Check sheet for the modelled part. Datum: model origin and axes. Units: mm. A direction names the side the tool comes from. Give positions to 0.01 mm unless a question says otherwise; leave off trailing zeros. Loops run counter-clockwise (first coordinate to the right, second up) from the corner with the lowest first, then second, coordinate; pieces in that order, holes last. Notation, with made-up numbers: M 57,-6.75 L 72,-6.75 A26 ccw 72,9.25 Z; hole C 4,-9.75 d2. An arc over 180 degrees is marked long. Use one line per item in the form item = value.
from build123d import *

# Parameters (mm, degrees)
EXTRUDE_1_DEPTH     = 20
SKETCH_2_R          = 2
CUT_EXTRUDE_1_DEPTH = 20
FILLET_1_R          = 2
FILLET_2_R          = 5
SKETCH_3_W          = 6.194211673
SKETCH_3_H          = 6.194211673
EXTRUDE_2_DEPTH     = 20


with BuildPart() as part:
    # 草图1 → 凸台-拉伸1 (new body)
    with BuildSketch(Plane.XY):
        Polygon((0, 0), (0, 50), (-5, 50), (-5, 35), (-25, 35), (-5, 15), (-5, 0), align=None)
    extrude(amount=EXTRUDE_1_DEPTH)

    # 草图2 → 切除-拉伸1 (cut)
    with BuildSketch(Plane.ZY.offset(5)):
        with Locations(Location((5, 42.5, 0), (0, 0, 270))):
            Circle(SKETCH_2_R)
        with Locations(Location((15, 42.5, 0), (0, 0, 270))):
            Circle(SKETCH_2_R)
        with Locations(Location((5, 7.5, 0), (0, 0, 270))):
            Circle(SKETCH_2_R)
        with Locations(Location((15, 7.5, 0), (0, 0, 270))):
            Circle(SKETCH_2_R)
    extrude(amount=-CUT_EXTRUDE_1_DEPTH, mode=Mode.SUBTRACT)

    # 圆角1
    fillet_1_edges = [part.edges().sort_by_distance(p)[0] for p in [
        (-5, 0, 10),
        (-5, 35, 10),
        (-5, 50, 10),
    ]]
    fillet(fillet_1_edges, radius=FILLET_1_R)

    # 圆角2
    fillet_2_edges = [part.edges().sort_by_distance(p)[0] for p in [
        (-5, 15, 10),
    ]]
    fillet(fillet_2_edges, radius=FILLET_2_R)

    # 草图3 → 凸台-拉伸2 (add, through all)
    with BuildSketch(Plane(origin=(0, 0, 0), x_dir=(-1, 0, 0), z_dir=(0, 0, -1))):
        with Locations((21.902894164, 31.902894164)):
            Rectangle(SKETCH_3_W, SKETCH_3_H)
    extrude(amount=-EXTRUDE_2_DEPTH)


solid = part.part
1) Section check C-C (z = 9). Record the cut outline in (x, y), then the cut area to 3 significant figures.
Evaluation:
outline = M -25,28.81 L -18.81,28.81 L -6.46,16.46 A5 cw -5,12.93 L -5,2 A2 ccw -3,0 L 0,0 L 0,50 L -3,50 A2 ccw -5,48 L -5,37 A2 cw -7,35 L -25,35 Z
area = 469 mm^2
2) Release check for a two-part mould opening along Z. For faces 1 (the face through (-5, 43, 10)), 2 (the face through (-8, 25, 0)), 3 (the face through (-2.535, 7.76, 16.983)), 4 (the face through (-8, 25, 20)) record: pulls with the +Z half, pulls with the -Z half, needs draft (parallel to the pull), parting line crosses it, or undercut.
Evaluation:
face_1 = needs draft
face_2 = pulls with the -Z half
face_3 = undercut
face_4 = pulls with the +Z half
3) Section check D-D (x = -8). Record the cut outline in (y, z), then the cut area to 3 significant figures.
Evaluation:
outline = M 18,0 L 35,0 L 35,20 L 18,20 Z
area = 340 mm^2
4) Set-up check for faces 5 (the face through (-16, 35, 10)), 6 (the face through (-5, 8, 10)), 7 (the face through (-2.535, 42.76, 16.983)): record each of +Z, -Z, +X, -X, +Y, -Y from which the full face is reachable in a straight line by a thin tool's end or side.
Evaluation:
face_5 = +Z, -Z, -X, +Y
face_6 = +Z, -Z, -X, -Y
face_7 = +X, -X
5) Section check A-A (z = 15). Record the cut outline in (x, y).
Evaluation:
outline = M -25,28.81 L -18.81,28.81 L -6.46,16.46 A5 cw -5,12.93 L -5,9.5 L 0,9.5 L 0,40.5 L -5,40.5 L -5,37 A2 cw -7,35 L -25,35 Z; M -5,2 A2 ccw -3,0 L 0,0 L 0,5.5 L -5,5.5 Z; M -5,44.5 L 0,44.5 L 0,50 L -3,50 A2 ccw -5,48 Z
6) Scan lines: line 1 (Z direction, x = -3, y = 7.5); line 2 (Y direction, x = -1.25, z = 16.25); line 3 (Z direction, x = -4, y = 44). Record each from-to range of solid material in increasing order.
Evaluation:
line_1 = 0 to 3, 7 to 13, 17 to 20
line_2 = 0 to 5.94, 9.06 to 40.94, 44.06 to 50
line_3 = 0 to 3.68, 6.32 to 13.68, 16.32 to 20
7) Depth check by flat-ended pin: pin 1 Ø6 at (y, z) = (25.5, 8) entering from -X; pin 2 Ø8.5 at (y, z) = (5.5, 13) entering from -X; pin 3 Ø3 at (x, z) = (-9.5, 5) entering from +Y; pin 4 Ø8 at (x, y) = (-6, 14) entering from +Z. Enter the tip coordinate at first touch or a pass-through.
Evaluation:
pin_1 = -18.5
pin_2 = -5
pin_3 = 35
pin_4 = 20
8) Section check B-B (y = 42.5). Record the cut outline in (x, z).
Evaluation:
outline = M -5,0 L 0,0 L 0,3 L -5,3 Z; M -5,7 L 0,7 L 0,13 L -5,13 Z; M -5,17 L 0,17 L 0,20 L -5,20 Z
